Print and shaded views of the part. All mm, measured from the part's lowest x, y and z. A direction names the side the tool comes from. Give positions to 0.01 mm unless a question says otherwise; leave off trailing zeros. Loops run counter-clockwise (first coordinate to the right, second up) from the corner with the lowest first, then second, coordinate; pieces in that order, holes last. Notation, with made-up numbers: (-15, -17) -> (-9, -17) arc R26 cw to (-9, 4) -> close; hole circle Ø2 at (-6, 11.25). An arc over 180 degrees is marked (long way). Write each question's results on one line, items separated by ' | '. Start each with the question number.
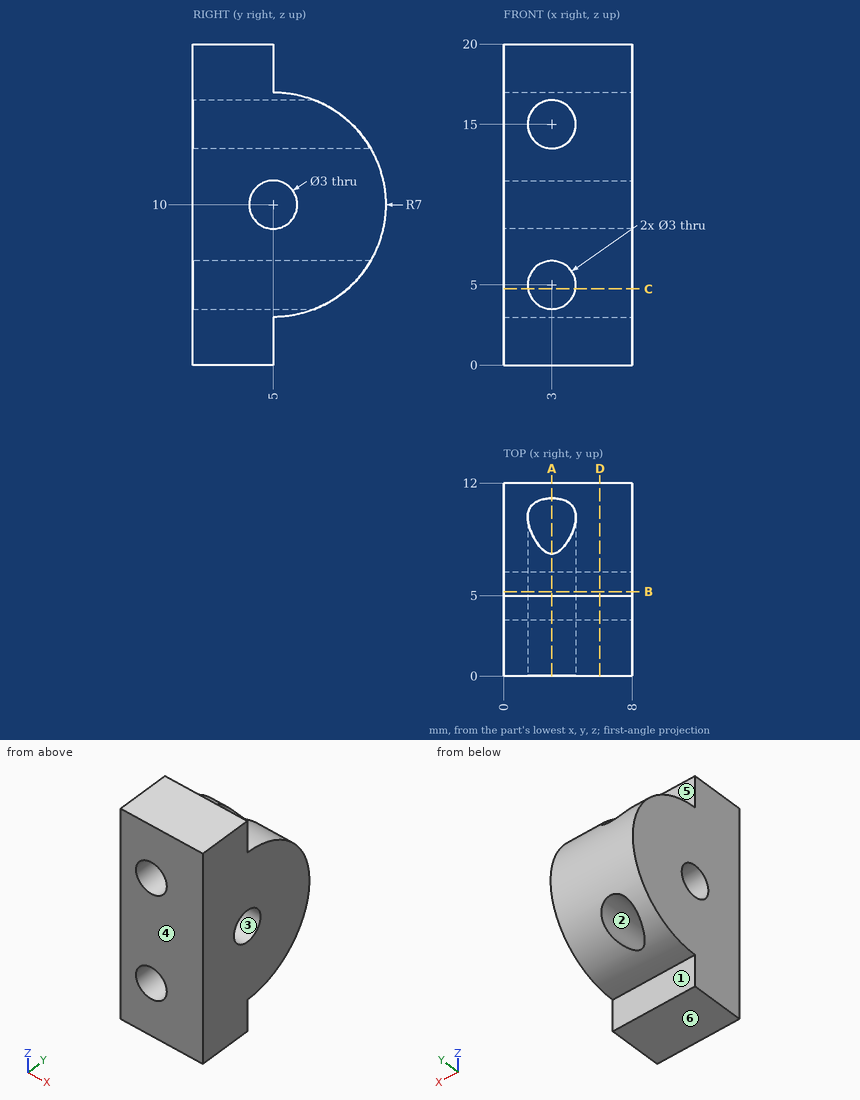
Q1. Mould opens along Y. For the marked faces 1, 2, 3 and 4 say: pulls with the +Y half, pulls with the -Y half, needs draft (parallel to the pull), parting line crosses it, or undercut.
Q2. Saw through at C-C, the plane z = 4.75. List the corners of the cut face in (x, y), then the cut area to 3 significant figures.
Q3. Saw through at B-B, the plane y = 5.25. List the corners of the cut face in (x, z).
Q4. Saw through at D-D, the plane x = 6. List the corners of the cut face in (y, z).
Q5. Saw through at A-A, the plane x = 3. List the corners of the cut face in (y, z), then the cut area to 3 significant figures.
Q6. Drop flat-ended pins along their axis: pin 1 (2.5 mm diameter, centred on x = 4.5, z = 19, fed in from +Y); pin 2 (2 mm diameter, centred on x = 4, z = 7, fed in from +Y). Give the stop position or say it passes through.
Q7. Wall check: L1, parallel to Y at x = 2, z = 10; L2, parallel to X at y = 3.5, z = 5; L3, parallel to Y at x = 5.75, z = 18.75. Give the ranges that are in metal, low to high.
Q8. Which spindle directions (+Z, -Z, +X, -X, +Y, -Y) get a long thin tool onto all of the face, cutting with end or side? Do the marked faces 5 and 6. Say none if no direction does.
Answer block:
1) face 1: pulls with the +Y half | face 2: needs draft | face 3: undercut | face 4: pulls with the -Y half
2) outline: (0, 0) -> (1.52, 0) -> (1.52, 9.63) -> (0, 9.63) -> close; (4.48, 0) -> (8, 0) -> (8, 9.63) -> (4.48, 9.63) -> close | area: 48.6 mm2
3) outline: (0, 3) -> (8, 3) -> (8, 8.52) -> (0, 8.52) -> close; (0, 11.48) -> (8, 11.48) -> (8, 17) -> (0, 17) -> close; hole circle Ø3 at (3, 5); hole circle Ø3 at (3, 15)
4) outline: (0, 0) -> (5, 0) -> (5, 3) arc R7 ccw to (5, 17) -> (5, 20) -> (0, 20) -> close; hole circle Ø3 at (5, 10)
5) outline: (0, 0) -> (5, 0) -> (5, 3) arc R7 ccw to (7.6, 3.5) -> (0, 3.5) -> close; (0, 6.5) -> (11.06, 6.5) arc R7 ccw to (11.06, 13.5) -> (0, 13.5) -> close; (0, 16.5) -> (7.6, 16.5) arc R7 ccw to (5, 17) -> (5, 20) -> (0, 20) -> close; hole circle Ø3 at (5, 10) | area: 112 mm2
6) pin 1: stops at y = 5 | pin 2: stops at y = 11.71
7) L1: y = 0 to 3.5, 6.5 to 12 | L2: x = 0 to 1.5, 4.5 to 8 | L3: y = 0 to 5
8) face 5: +Z, +X, -X, +Y | face 6: -Z, +X, -X, +Y, -Y
